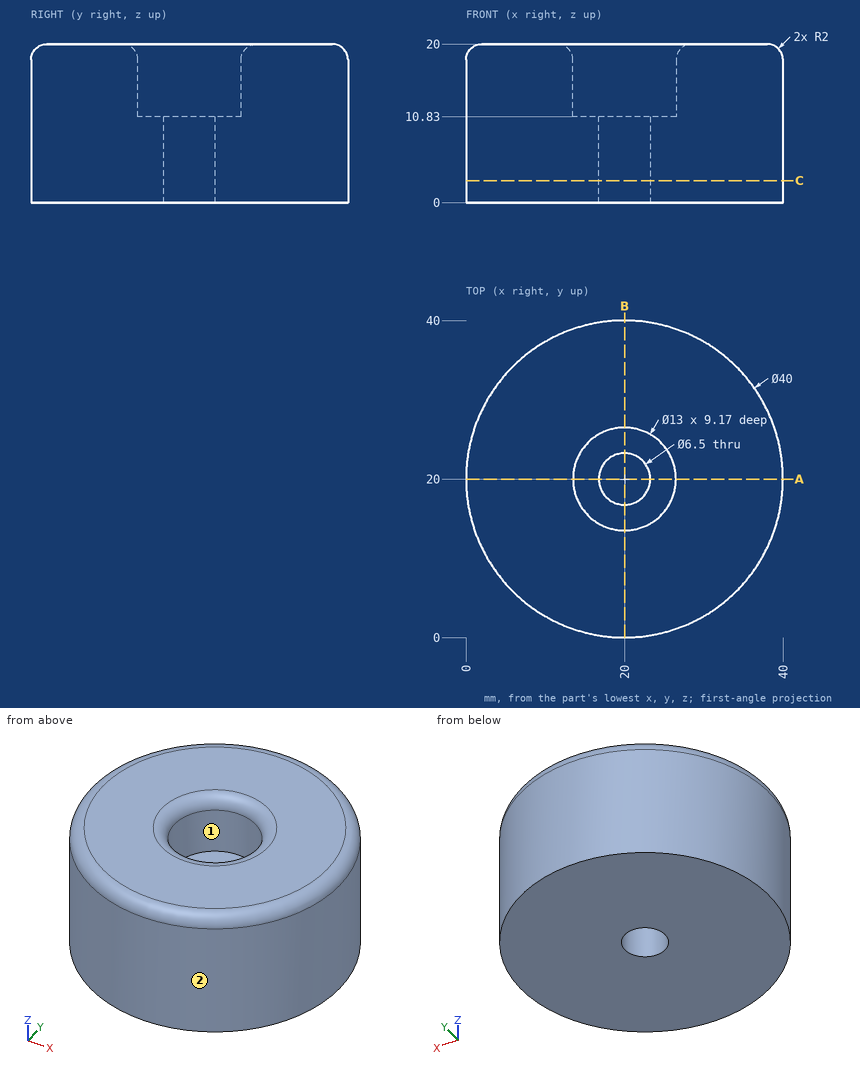
The drawing under review shows one solid part. Ordinate dimensions are in mm from its lowest x, y, z. A direction names the side the tool comes from. Coordinates: 2 decimals unless noted, no trailing zeros. Order: outer loops, then holes, each group sorted by start corner. A loop starts at its lowest first (then second) coordinate and runs counter-clockwise, first axis right, second up. Notation, with made-up numbers: (-23, 38) -> (13, 38) arc R32 ccw to (13, 67) -> close; hole circle Ø3 at (10, 64). An arc over 180 degrees is marked (long way). Return JSON: item names as keys, results as strings.
1. Machinability: for the marked faces 1 and 2, which of the approach directions +Z, -Z, +X, -X, +Y, -Y give a long, thin tool a straight path to every point of the face, cutting with its end or side? Answer none if there is none.
Answer block:
{"face 1": "+Z", "face 2": "+Z, -Z"}
2. For line 1 (Y direction, x = 20, z = 8.5); line 2 (Y direction, x = 20, z = 16); line 3 (Z direction, x = 18, y = 23), list the stretches that pass through material, from the lowest coordinate up. Write a range as from..to.
Answer block:
{"line 1": "0..16.75, 23.25..40", "line 2": "0..13.5, 26.5..40", "line 3": "0..10.83"}
3. We need section A-A on y = 20. Write out the cut boundary in (x, z), and give its area (3 significant figures).
Answer block:
{"outline": "(0, 0) -> (16.75, 0) -> (16.75, 10.83) -> (13.5, 10.83) -> (13.5, 18) arc R2 ccw to (11.5, 20) -> (2, 20) arc R2 ccw to (0, 18) -> close; (23.25, 0) -> (40, 0) -> (40, 18) arc R2 ccw to (38, 20) -> (28.5, 20) arc R2 ccw to (26.5, 18) -> (26.5, 10.83) -> (23.25, 10.83) -> close", "area": "607 mm²"}
4. For pin 1 Ø2 at (y, z) = (14, 5.5) entering from +X; pin 2 Ø4 at (x, z) = (15, 8.5) entering from +Y; pin 3 Ø12 at (x, z) = (31.5, 15.5) entering from -Y, all flat-tipped, find the tip position at first contact; note any pin that passes through.
Answer block:
{"pin 1": "x = 39.36", "pin 2": "y = 39.77", "pin 3": "y = 0.77"}
5. We need section C-C on z = 2.75. Write out the cut boundary in (x, y), and give its area (3 significant figures).
Answer block:
{"outline": "circle Ø40 at (20, 20); hole circle Ø6.5 at (20, 20)", "area": "1,220 mm²"}
